Verification items for the finished model (mm, model axes). Face numbers are marked on the shaded views. A direction names the side the tool comes from. Round coordinates to 2 decimals unless told otherwise and drop trailing zeros. Loops run counter-clockwise (first coordinate to the right, second up) from the corner with the lowest first, then second, coordinate; pieces in that order, holes last. Notation, with made-up numbers: M 15.25,-20 L 61.25,-20 A22 cw 61.25,8 Z; hole C -18.5,-17.75 d10. An arc over 180 degrees is marked long. One line per item, written item: value.
from build123d import *

# Parameters (mm, degrees)
SKETCH1_W           = 210
SKETCH1_H           = 75
BOSS_EXTRUDE1_DEPTH = 4
SKETCH2_W           = 210
SKETCH2_H           = 4
BOSS_EXTRUDE2_DEPTH = 60
SKETCH3_W           = 4
SKETCH3_H           = 71
BOSS_EXTRUDE3_DEPTH = 30
FILLET1_R           = 10
SKETCH5_W           = 4
SKETCH5_H           = 61
BOSS_EXTRUDE4_DEPTH = 20


with BuildPart() as part:
    # Sketch1 → Boss-Extrude1 (new body)
    with BuildSketch(Plane.XY):
        with Locations((-9.965753425, 81.934931507)):
            Rectangle(SKETCH1_W, SKETCH1_H)
    extrude(amount=BOSS_EXTRUDE1_DEPTH)

    # Sketch2 → Boss-Extrude2 (add)
    with BuildSketch(Plane.XY):
        with Locations((-9.965753425, 46.434931507)):
            Rectangle(SKETCH2_W, SKETCH2_H)
    extrude(amount=-BOSS_EXTRUDE2_DEPTH)

    # Sketch3 → Boss-Extrude3 (add)
    with BuildSketch(Plane.XY):
        with Locations((-112.965753425, 83.934931507)):
            Rectangle(SKETCH3_W, SKETCH3_H)
        with Locations((93.034246575, 83.934931507)):
            Rectangle(SKETCH3_W, SKETCH3_H)
    extrude(amount=-BOSS_EXTRUDE3_DEPTH)

    # Fillet1
    # the kernel refuses this fillet: 10 mm, written as the material it takes off along each edge
    with BuildSketch(Plane(origin=(-110.965753425, 119.434931507, 0), x_dir=(0, 0, 1), z_dir=(1, 0, 0))) as fillet1_piece_1:
        with BuildLine():
            CenterArc((FILLET1_R, FILLET1_R), FILLET1_R, 180, 90)
            Line((0, FILLET1_R), (0, 0))
            Line((0, 0), (FILLET1_R, 0))
        make_face()
    extrude(amount=202, mode=Mode.SUBTRACT)

    # Sketch5 → Boss-Extrude4 (add)
    with BuildSketch(Plane(origin=(0, 0, 0), x_dir=(-1, 0, 0), z_dir=(0, 0, -1))):
        with Locations((9.965753425, 78.934931507)):
            Rectangle(SKETCH5_W, SKETCH5_H)
    extrude(amount=BOSS_EXTRUDE4_DEPTH)


solid = part.part
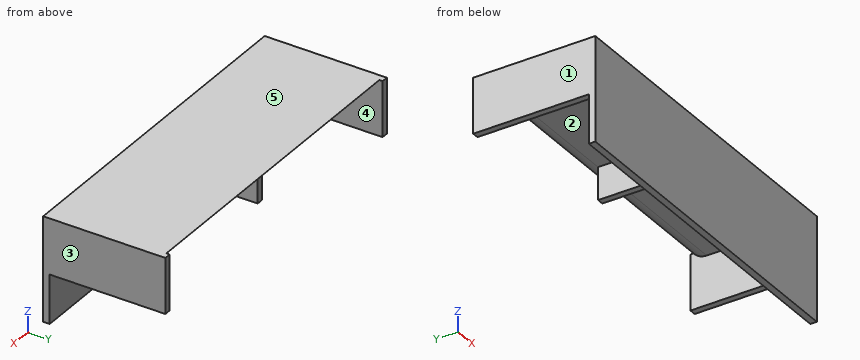
(1) Thickness scan on L1, parallel to X at y = 105.5, z = -4; L2, parallel to X at y = 48.5, z = -29.5; L3, parallel to Y at x = -35, z = -43. Record the ranges inside material, lowest first. Write a range as from..to.
Completed:
L1: x = -114.97..-110.97, -11.97..-7.97, 91.03..95.03
L2: x = -114.97..-110.97, 91.03..95.03
L3: y = 44.43..48.43
(2) Sectioned sample at D-D on z = -23. Enter the section's corners in (x, y), and give its area (3 significant figures).
Completed:
outline: M -114.97,44.43 L 95.03,44.43 L 95.03,119.43 L 91.03,119.43 L 91.03,48.43 L -110.97,48.43 L -110.97,119.43 L -114.97,119.43 Z
area: 1,410 mm^2
(3) Sectioned sample at C-C on y = 65. Enter the section's corners in (x, z).
Completed:
outline: M -114.97,-30 L -110.97,-30 L -110.97,0 L -11.97,0 L -11.97,-20 L -7.97,-20 L -7.97,0 L 91.03,0 L 91.03,-30 L 95.03,-30 L 95.03,4 L -114.97,4 Z
(4) Sectioned sample at B-B on z = -7. Enter the section's corners in (x, y).
Completed:
outline: M -114.97,44.43 L 95.03,44.43 L 95.03,119.43 L 91.03,119.43 L 91.03,48.43 L -7.97,48.43 L -7.97,109.43 L -11.97,109.43 L -11.97,48.43 L -110.97,48.43 L -110.97,119.43 L -114.97,119.43 Z
(5) Depth check by flat-ended pin: pin 1 Ø1.2 at (x, y) = (-112.5, 88) entering from -Z; pin 2 Ø1 at (x, z) = (-53.5, -30) entering from +Y; pin 3 Ø12 at (x, y) = (41, 91) entering from -Z. Enter the tip coordinate at first touch or a pass-through.
Completed:
pin 1: stops at z = -30
pin 2: stops at y = 48.43
pin 3: stops at z = 0
(6) Tool access check on the marked faces 4 and 5. Record the directions out of +Z, -Z, +X, -X, +Y, -Y that give a thin tool (end or side, any length) a straight path to the whole face; none if there is none.
Completed:
face 4: -Z, +Y
face 5: +Z, +X, -X, +Y, -Y
(7) Sectioned sample at A-A on x = -64.5. Enter the section's corners in (y, z).
Completed:
outline: M 44.43,-60 L 48.43,-60 L 48.43,0 L 109.43,0 A10 ccw 117.43,4 L 44.43,4 Z
(8) Mould release check, pull along X, two halves, no side actions. Record for the marked faces 1, 2 and 3: +X half, -X half, draft (parallel to the pull), parting line (faces both ways), or undercut.
Completed:
face 1: -X half
face 2: undercut
face 3: +X half
